from build123d import *

# Parameters (mm, degrees)
SKETCH1_W               = 40
SKETCH1_H               = 40
SKETCH1_W_2             = 20.4
SKETCH1_H_2             = 20.4
BOSS_EXTRUDE1_DEPTH     = 80
SKETCH1_2_W             = 40
SKETCH1_2_H             = 40
SKETCH1_2_W_2           = 20.4
SKETCH1_2_H_2           = 20.4
BOSS_EXTRUDE2_DEPTH     = 30
CUT_EXTRUDE1_DEPTH      = 91.68671347
CUT_EXTRUDE1_DEPTH_BACK = 91.68671347
SKETCH2_R               = 2.75
SKETCH3_R               = 5.15
CUT_EXTRUDE4_DEPTH      = 95.403601626
FILLET1_R               = 5
CUT_EXTRUDE6_DEPTH      = 10.5
CUT_EXTRUDE7_DEPTH      = 20
FILLET2_R               = 5


with BuildPart() as part:
    # Sketch1 → Boss-Extrude1 (new body)
    with BuildSketch(Plane(origin=(0, 0, 0), x_dir=(1, 0, 0), z_dir=(0, 1, 0))):
        with Locations((10.2, 10.2)):
            Rectangle(SKETCH1_W, SKETCH1_H)
        with Locations((10.2, 10.2)):
            Rectangle(SKETCH1_W_2, SKETCH1_H_2, mode=Mode.SUBTRACT)
    extrude(amount=BOSS_EXTRUDE1_DEPTH)

    # Sketch1_2 → Boss-Extrude2 (add)
    # profile 1 of 2: a face of its own
    with BuildSketch(Plane(origin=(0, 0, 0), x_dir=(1, 0, 0), z_dir=(0, 1, 0))):
        with Locations((10.2, 10.2)):
            Rectangle(SKETCH1_2_W, SKETCH1_2_H)
        with Locations((10.2, 10.2)):
            Rectangle(SKETCH1_2_W_2, SKETCH1_2_H_2, mode=Mode.SUBTRACT)
    # profile 2 of 2: a face of its own
    with BuildSketch(Plane(origin=(0, 0, 0), x_dir=(1, 0, 0), z_dir=(0, 1, 0))):
        with Locations((10.2, 10.2)):
            Rectangle(SKETCH1_2_W_2, SKETCH1_2_H_2)
    extrude(amount=-BOSS_EXTRUDE2_DEPTH)

    # Sketch2 → Cut-Extrude1 (cut, two sides: drawn at the far end of the back side and taken through both)
    with BuildSketch(Plane(origin=(0, 0, 0), x_dir=(-1, 0, 0), z_dir=(0, 0, -1)).offset(-CUT_EXTRUDE1_DEPTH_BACK)):
        with Locations((-10.2, 15)):
            Circle(SKETCH2_R)
        with Locations((-10.2, 65)):
            Circle(SKETCH2_R)
    extrude(amount=CUT_EXTRUDE1_DEPTH + CUT_EXTRUDE1_DEPTH_BACK, mode=Mode.SUBTRACT)

    # Sketch3 → Cut-Extrude4 (cut, through all)
    with BuildSketch(Plane.ZY.offset(9.8)):
        with Locations((-10.2, -15)):
            Circle(SKETCH3_R)
    extrude(amount=-CUT_EXTRUDE4_DEPTH, mode=Mode.SUBTRACT)

    # Fillet1
    fillet1_edges = [part.edges().sort_by_distance(p)[0] for p in [
        (-9.8, 25, -30.2),
        (30.2, 25, -30.2),
        (30.2, 25, 9.8),
        (-9.8, 25, 9.8),
    ]]
    fillet(fillet1_edges, radius=FILLET1_R)

    # Sketch4 → Cut-Extrude6 (cut)
    with BuildSketch(Plane.XY.offset(9.8)):
        with BuildLine():
            ThreePointArc((7.45, -15), (10.2, -17.75), (12.95, -15))
            Line((12.95, -15), (7.45, -15))
        make_face()
        with BuildLine():
            Line((7.45, -15), (12.95, -15))
            ThreePointArc((12.95, -15), (10.2, -12.25), (7.45, -15))
        make_face()
        with BuildLine():
            ThreePointArc((7.1, -15), (10.2, -18.1), (13.3, -15))
            Line((13.3, -15), (12.95, -15))
            ThreePointArc((12.95, -15), (10.2, -17.75), (7.45, -15))
            Line((7.45, -15), (7.1, -15))
        make_face()
        with BuildLine():
            Line((12.95, -15), (13.3, -15))
            ThreePointArc((13.3, -15), (10.2, -11.9), (7.1, -15))
            Line((7.1, -15), (7.45, -15))
            ThreePointArc((7.45, -15), (10.2, -12.25), (12.95, -15))
        make_face()
    extrude(amount=-CUT_EXTRUDE6_DEPTH, mode=Mode.SUBTRACT)

    # Sketch4_3 → Cut-Extrude7 (cut)
    with BuildSketch(Plane.XY.offset(9.8)):
        with BuildLine():
            ThreePointArc((7.45, -15), (10.2, -17.75), (12.95, -15))
            Line((12.95, -15), (7.45, -15))
        make_face()
        with BuildLine():
            Line((7.45, -15), (12.95, -15))
            ThreePointArc((12.95, -15), (10.2, -12.25), (7.45, -15))
        make_face()
    extrude(amount=-CUT_EXTRUDE7_DEPTH, mode=Mode.SUBTRACT)

    # Fillet2
    fillet2_edges = [part.edges().sort_by_distance(p)[0] for p in [
        (-9.8, 80, -10.2),
        (10.2, 80, -30.2),
        (10.2, 80, 9.8),
        (30.2, 80, -10.2),
        (28.735533906, 80, -28.735533906),
        (28.735533906, 80, 8.335533906),
        (-8.335533906, 80, 8.335533906),
        (-8.335533906, 80, -28.735533906),
    ]]
    fillet(fillet2_edges, radius=FILLET2_R)


solid = part.part
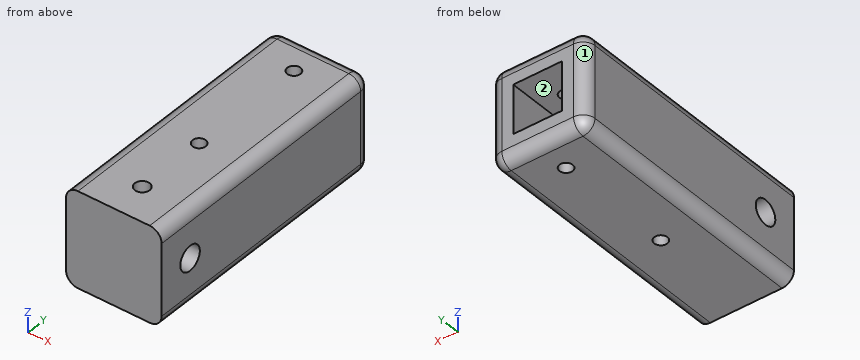
Source: CAD feature listing. Evaluate the final solid. Frame: model axes, mm. Face numbers are marked on the shaded views. A direction names the side the tool comes from. Give positions to 0.01 mm unless a question says otherwise; leave off trailing zeros. Write each loop counter-clockwise with the first axis right and the second up, starting at its lowest first coordinate (ties: lowest second). Pieces come first, ordered by that corner, then holes. Notation, with made-up numbers: M 72.25,7 L 86.25,7 A27 cw 86.25,38 Z; hole C 34,-16.5 d2. An arc over 180 degrees is marked long. Return JSON: item names as keys, results as strings. Group by question number.
1) Cut plane A-A, the plane y = 15. Output: boundary loops of the cut face in (x, z), plus the area to 3 significant figures.
2) Set-up query: the marked faces 1 and 2. Return all of +Z, -Z, +X, -X, +Y, -Y with unobstructed straight access to the full face (end or side cutting, diameter ignored); none if empty.
3) Material intervals for line 1 along Y through (x, z) = (10.2, -24); line 2 along Y through (x, z) = (10.2, 4); line 3 along Y through (x, z) = (10, -26), sorted ascending. Write a range as [from, to].
4) Pin query (flat end, axial travel): P1, Ø5, axis at x = 10, y = -15, coming from the +Z side; P2, Ø5, axis at x = 10.2, y = 65, coming from the -Z side; P3, Ø10, axis at x = 12, z = -12, coming from the +Y side; P4, Ø4.5, axis at x = 10.2, y = -15, coming from the +Z side. Return the tip coordinate at first contact, or that it passes through.
5) Cut plane B-B, the plane x = -1.5. Output: boundary loops of the cut face in (y, z).
6) Cut plane C-C, the plane y = -15. Output: boundary loops of the cut face in (x, z), plus the area to 3 significant figures.
7) Cut plane D-D, the plane z = 1. Output: boundary loops of the cut face in (x, y).
Recorded:
{
 "1": {"outline": "M -9.8,-25.2 A5 ccw -4.8,-30.2 L 7.45,-30.2 L 7.45,-20.4 L 0,-20.4 L 0,0 L 7.45,0 L 7.45,9.8 L -4.8,9.8 A5 ccw -9.8,4.8 Z; M 12.95,-30.2 L 25.2,-30.2 A5 ccw 30.2,-25.2 L 30.2,4.8 A5 ccw 25.2,9.8 L 12.95,9.8 L 12.95,0 L 20.4,0 L 20.4,-20.4 L 12.95,-20.4 Z", "area": "1,050 mm²"},
 "2": {"face 1": "+Z, -Z, -X, +Y", "face 2": "+Y"},
 "3": {"line 1": "y = [-30, 12.25], [17.75, 62.25], [67.75, 80]", "line 2": "y = [-30, -18.1], [-11.9, 12.25], [17.75, 62.25], [67.75, 80]", "line 3": "y = [-30, 12.26], [17.74, 62.26], [67.74, 79.94]"},
 "4": {"P1": "stops at z = -14.7", "P2": "passes through", "P3": "stops at y = 0", "P4": "stops at z = -14.83"},
 "5": {"outline": "M -30,-30.2 L 75,-30.2 A5 ccw 80,-25.2 L 80,4.8 A5 ccw 75,9.8 L -30,9.8 Z; hole C -15,-10.2 d10.3"},
 "6": {"outline": "M -9.8,-25.2 A5 ccw -4.8,-30.2 L 25.2,-30.2 A5 ccw 30.2,-25.2 L 30.2,-15.35 L -9.8,-15.35 Z; M -9.8,-5.05 L 7.45,-5.05 L 7.45,-0.7 L 7.1,-0.7 L 7.1,9.8 L -4.8,9.8 A5 ccw -9.8,4.8 Z; M 12.95,-5.05 L 30.2,-5.05 L 30.2,4.8 A5 ccw 25.2,9.8 L 13.3,9.8 L 13.3,-0.7 L 12.95,-0.7 Z", "area": "1,080 mm²"},
 "7": {"outline": "M -9.8,-30 L 30.2,-30 L 30.2,75 A5 ccw 25.2,80 L -4.8,80 A5 ccw -9.8,75 Z; hole C 10.2,-15 d6.2; hole C 10.2,15 d5.5; hole C 10.2,65 d5.5"}
}
